```python
from build123d import *

# Parameters (mm, degrees)
F1_DEPTH = 10
F2_R     = 1
F4_R     = 5.5
F5_DEPTH = 113.001
F7_R     = 3.5
F8_DEPTH = 90.501
F9_R     = 1
F10_R    = 1


with BuildPart() as f1:
    # F0 (on Front) → F1 (new body, symmetric)
    with BuildSketch(Plane.XZ):
        with BuildLine():
            Line((-56.5, 65.5), (-56.5, 50.5))
            ThreePointArc((-56.5, 50.5), (0, -6), (56.5, 50.5))
            Line((56.5, 50.5), (56.5, 65.5))
            Line((56.5, 65.5), (50.5000007153, 65.5))
            Line((50.5000007153, 65.5), (50.5000007153, 50.5))
            ThreePointArc((50.5000007153, 50.5), (7.153e-07, 0), (-50.4999992847, 50.5))
            Line((-50.4999992847, 50.5), (-50.4999992847, 65.5))
            Line((-50.4999992847, 65.5), (-56.5, 65.5))
        make_face()
    extrude(amount=F1_DEPTH, both=True)

    # F2
    f2_edges = [f1.edges().sort_by_distance(p)[0] for p in [
        (1e-06, -10, 0),
        (-50.499999, -10, 58),
        (50.500001, -10, 58),
        (0, -10, -6),
        (-56.5, -10, 58),
        (-50.499999, 10, 58),
        (1e-06, 10, 0),
        (50.500001, 10, 58),
        (56.5, 10, 58),
        (0, 10, -6),
        (-56.5, 10, 58),
    ]]
    fillet(f2_edges, radius=F2_R)

    # F4 (on offset) → F5 (cut, through all)
    with BuildSketch(Plane.YZ.offset(56.5)):
        with Locations((0, 57.9845793545)):
            Circle(F4_R)
    extrude(amount=-F5_DEPTH, mode=Mode.SUBTRACT)

    # F7 (on offset) → F8 (cut, through all)
    with BuildSketch(Plane.XY.offset(-25)):
        Circle(F7_R)
    extrude(amount=F8_DEPTH, mode=Mode.SUBTRACT)

    # F9
    f9_edges = [f1.edges().sort_by_distance(p)[0] for p in [
        (-50.499999, 0, 65.5),
        (-50.792893, -9.707107, 65.5),
        (-53.5, -10, 65.5),
        (-56.5, 0, 65.5),
        (-56.207107, -9.707107, 65.5),
        (-56.207107, 9.707107, 65.5),
        (-53.5, 10, 65.5),
        (-50.792893, 9.707107, 65.5),
    ]]
    fillet(f9_edges, radius=F9_R)

    # F10
    f10_edges = [f1.edges().sort_by_distance(p)[0] for p in [
        (56.5, 0, 65.5),
        (56.207107, -9.707107, 65.5),
        (53.5, -10, 65.5),
        (50.792894, -9.707107, 65.5),
        (50.500001, 0, 65.5),
        (50.792894, 9.707107, 65.5),
        (53.5, 10, 65.5),
        (56.207107, 9.707107, 65.5),
    ]]
    fillet(f10_edges, radius=F10_R)


solid = f1.part
```
Check sheet for the modelled part. Datum: model origin and axes. Units: mm. A direction names the side the tool comes from. Round coordinates to 2 decimals unless told otherwise and drop trailing zeros. Order: outer loops, then holes, each group sorted by start corner. A loop starts at its lowest first (then second) coordinate and runs counter-clockwise, first axis right, second up. Notation, with made-up numbers: M 1,41 L 36,41 A14 cw 36,64 Z; hole C -6.5,35 d7. An arc over 180 degrees is marked long. Answer in a Markdown table with one row per item.
(1) Gauge pin test, flat ends, axial feed: pin 1 (6 mm diameter, centred on x = -32.5, y = 8, fed in from -Z); pin 2 (3 mm diameter, centred on x = 9, y = 6, fed in from -Z); pin 3 (4 mm diameter, centred on y = 2, z = 56.5, fed in from -X); pin 4 (4 mm diameter, centred on y = -5, z = 8, fed in from -X). Record the tip position at first contact, or that the pin passes through.
Findings:
| item | result |
|---|---|
| pin 1 | stops at z = 2.31 |
| pin 2 | stops at z = -5.5 |
| pin 3 | passes through |
| pin 4 | stops at x = -39.4 |
(2) Draft check along Y on faces 1 (the flat face through (-50.5, -2.1, 52.7)), 2 (the cylindrical face through (-53.458, -0.716, 63.438)), 3 (the flat face through (4, -10, -1)). Enter one of: +Y half, -Y half, draft (parallel to the pull), parting line (faces both ways), or undercut.
Findings:
| item | result |
|---|---|
| face 1 | draft |
| face 2 | undercut |
| face 3 | -Y half |
(3) Material ranges on line 1 along X through (y, z) = (9, 58); line 2 along Y through (x, z) = (0, -2.25); line 3 along Y through (x, z) = (-43, 22.5), recorded low to high. Write a range as from..to.
Findings:
| item | result |
|---|---|
| line 1 | x = -56.5..-50.5, 50.5..56.5 |
| line 2 | y = -10..-3.5, 3.5..10 |
| line 3 | y = -9.98..9.98 |
(4) Set-up check for faces 4 (the cylindrical face through (3.233, -1.341, -2.984)), 5 (the flat face through (50.5, 6, 58)): record each of +Z, -Z, +X, -X, +Y, -Y from which the full face is reachable in a straight line by a thin tool's end or side.
Findings:
| item | result |
|---|---|
| face 4 | +Z, -Z |
| face 5 | +Z, +Y, -Y |
(5) Section check A-A on y = 0. Record the boundary of the cut face in (x, z).
Findings:
| item | result |
|---|---|
| outline | M -56.5,50.5 A56.5 ccw -3.5,-5.89 L -3.5,0.12 A50.5 cw -50.5,50.5 L -50.5,52.48 L -56.5,52.48 Z; M -56.5,63.48 L -50.5,63.48 L -50.5,64.5 A1 ccw -51.5,65.5 L -55.5,65.5 A1 ccw -56.5,64.5 Z; M 3.5,-5.89 A56.5 ccw 56.5,50.5 L 56.5,52.48 L 50.5,52.48 L 50.5,50.5 A50.5 cw 3.5,0.12 Z; M 50.5,63.48 L 56.5,63.48 L 56.5,64.5 A1 ccw 55.5,65.5 L 51.5,65.5 A1 ccw 50.5,64.5 Z |
